Design review of the part built by this model. Coordinates are the model's own, in mm. Face numbers are marked on the shaded views. A direction names the side the tool comes from. Give positions to 0.01 mm unless a question says otherwise; leave off trailing zeros. Order: outer loops, then holes, each group sorted by start corner. A loop starts at its lowest first (then second) coordinate and runs counter-clockwise, first axis right, second up. Notation, with made-up numbers: M -15.5,51.25 L 12.5,51.25 A24 cw 12.5,64.25 Z; hole C 18,89 d8. An arc over 180 degrees is marked long. Answer as a JSON object with one key per item and string values.
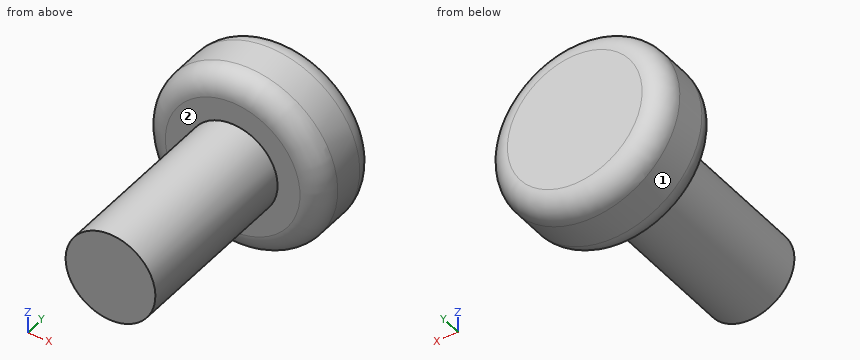
from build123d import *

# Parameters (mm, degrees)
FILLET1_R = 0.5


with BuildPart() as part:
    # Sketch1 → Revolve1 (revolve)
    with BuildSketch(Plane.XY, mode=Mode.PRIVATE) as revolve1_sk:
        Polygon((0, 0), (-1, 0), (-1, 4), (-2, 4), (-2, 5.72), (0, 5.72), align=None)
    revolve(revolve1_sk.sketch.rotate(Axis((0, 5.72, 0), (0, -1, 0)), 270), axis=Axis((0, 5.72, 0), (0, -1, 0)))

    # Fillet1
    fillet1_edges = [part.edges().sort_by_distance(p)[0] for p in [
        (0, 5.72, -2),
        (0, 4, -2),
    ]]
    fillet(fillet1_edges, radius=FILLET1_R)


solid = part.part
(1) Insertion check: pin 1 (2 mm diameter, centred on x = 1, y = 1, fed in from +Z); pin 2 (1 mm diameter, centred on x = -1, y = 5, fed in from +Z); pin 3 (2 mm diameter, centred on y = 1, z = 0, fed in from -X). Each pin has a flat end and moves straight along its axis. Give the tip position at first contact, or say it passes through.
Checked values:
{"pin 1": "stops at z = 1", "pin 2": "stops at z = 1.94", "pin 3": "stops at x = -1"}
(2) We need section B-B (x = 0). Write out the cut boundary in (y, z).
Checked values:
{"outline": "M 0,-1 L 4,-1 L 4,-1.5 A0.5 ccw 4.5,-2 L 5.22,-2 A0.5 ccw 5.72,-1.5 L 5.72,1.5 A0.5 ccw 5.22,2 L 4.5,2 A0.5 ccw 4,1.5 L 4,1 L 0,1 Z"}
(3) Tool access review of the marked faces 1 and 2: name each direction out of +Z, -Z, +X, -X, +Y, -Y from which nothing blocks a thin tool from reaching the whole face with its end or side.
Checked values:
{"face 1": "+Y, -Y", "face 2": "-Y"}
(4) To check wall thickness, follow L1, parallel to Y at x = 1.4, z = 0.35; L2, parallel to Z at x = -0.75, y = 4.4; L3, parallel to X at y = 1.35, z = -0.5. State the ranges of each line that lie inside material, in increasing order. Write a range as from..to.
Checked values:
{"L1": "y = 4..5.72", "L2": "z = -1.84..1.84", "L3": "x = -0.87..0.87"}
(5) We need section C-C (y = 4.2). Write out the cut boundary in (x, z).
Checked values:
{"outline": "C 0,0 d3.8"}
(6) We need section D-D (y = 0.9). Write out the cut boundary in (x, z).
Checked values:
{"outline": "C 0,0 d2"}
(7) We need section A-A (z = 0). Write out the cut boundary in (x, y), plus the area to 3 significant figures.
Checked values:
{"outline": "M -2,4.5 A0.5 ccw -1.5,4 L -1,4 L -1,0 L 1,0 L 1,4 L 1.5,4 A0.5 ccw 2,4.5 L 2,5.22 A0.5 ccw 1.5,5.72 L -1.5,5.72 A0.5 ccw -2,5.22 Z", "area": "14.7 mm^2"}
